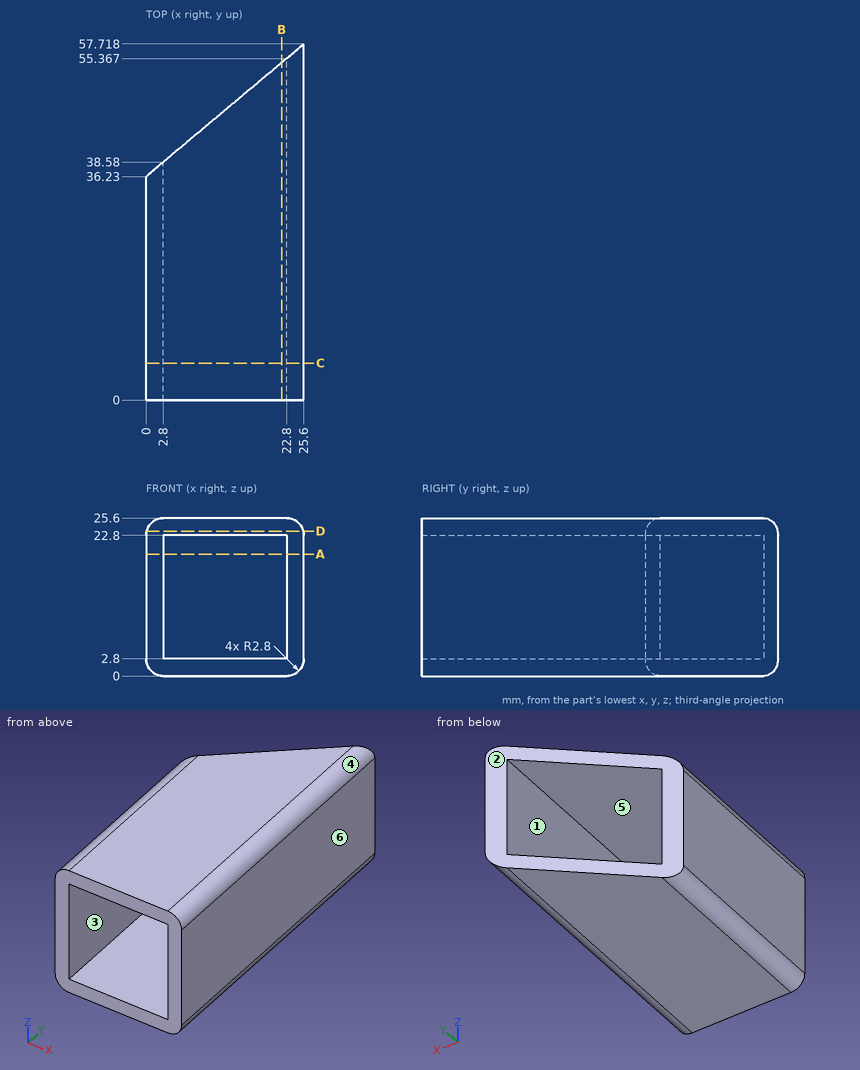
Input: dimensioned drawing with shaded views. Units: mm. Origin: part minimum x, y, z. A direction names the side the tool comes from. Coordinates: 2 decimals unless noted, no trailing zeros. Loops run counter-clockwise (first coordinate to the right, second up) from the corner with the lowest first, then second, coordinate; pieces in that order, holes last. Notation, with made-up numbers: M 38.25,25.5 L 53.25,25.5 A30 ccw 53.25,51.5 Z; hole C 89.25,61 d11. An arc over 180 degrees is marked long. Use a Markdown table: item, result. Add a question column.
Q1. Material intervals for L1, parallel to Z at x = 4, y = 8.5; L2, parallel to X at y = 43, z = 9.5, sorted ascending.
Q2. Access query for the marked faces 5 and 6. Directions: +Z, -Z, +X, -X, +Y, -Y. A direction counts if a zero-diameter tool reaches every point of the face in a straight line with its end or side. Return the directions, or none.
Q3. Section query B-B, the plane x = 22. Return loops of the section in (y, z).
Q4. Section query C-C, the plane y = 6. Return loops of the section in (x, z).
Q5. Section query D-D, the plane z = 23.5. Return loops of the section in (x, y) (1 decimal).
Q6. First-contact query: pin 1 (5 mm diameter, centred on x = 8, z = 19.5, fed in from +Y). Flat tip, straight axial feed; report the tip coordinate or a pass-through.
Q7. Draft query along X for the marked faces 1, 2, 3 and 4. Return one class per face: pulls with the +X half, pulls with the -X half, needs draft (parallel to the pull), parting line crosses it, or undercut.
Q8. Section query A-A, the plane z = 19.75. Return loops of the section in (x, y), and give its area (3 significant figures).
Result:
| question | item | result |
|---|---|---|
| 1 | L1 | z = 0 to 2.8, 22.8 to 25.6 |
| 1 | L2 | x = 22.8 to 25.6 |
| 2 | face 5 | +Y, -Y |
| 2 | face 6 | +Z, -Z, +X, +Y, -Y |
| 3 | outline | M 0,0 L 54.7,0 L 54.7,2.8 L 0,2.8 Z; M 0,22.8 L 54.7,22.8 L 54.7,25.6 L 0,25.6 Z |
| 4 | outline | M 0,2.8 A2.8 ccw 2.8,0 L 22.8,0 A2.8 ccw 25.6,2.8 L 25.6,22.8 A2.8 ccw 22.8,25.6 L 2.8,25.6 A2.8 ccw 0,22.8 Z; hole M 2.8,2.8 L 22.8,2.8 L 22.8,22.8 L 2.8,22.8 Z |
| 5 | outline | M 0.1,0 L 25.5,0 L 25.5,57.6 L 0.1,36.3 Z |
| 6 | pin 1 | passes through |
| 7 | face 1 | undercut |
| 7 | face 2 | pulls with the -X half |
| 7 | face 3 | undercut |
| 7 | face 4 | pulls with the +X half |
| 8 | outline | M 0,0 L 2.8,0 L 2.8,38.58 L 0,36.23 Z; M 22.8,0 L 25.6,0 L 25.6,57.72 L 22.8,55.37 Z |
| 8 | area | 263 mm2 |
